Model file for the job. Use its own axes, mm. Face numbers are marked on the shaded views. A direction names the side the tool comes from. Round coordinates to 2 decimals unless told otherwise and drop trailing zeros. Loops run counter-clockwise (first coordinate to the right, second up) from the corner with the lowest first, then second, coordinate; pieces in that order, holes last. Notation, with made-up numbers: (44, 6) -> (70, 6) arc R14 cw to (70, 24) -> close; hole circle Ø7 at (58, 82). An arc over 180 degrees is marked (long way). Use a Markdown table: item, result.
from build123d import *

# Parameters (mm, degrees)
SKETCH_8_W      = 120
SKETCH_8_H      = 120
SKETCH_8_W_2    = 100
SKETCH_8_H_2    = 100
EXTRUDE_1_DEPTH = 225
SKETCH_9_W      = 160
SKETCH_9_H      = 160
SKETCH_9_R      = 25
EXTRUDE_2_DEPTH = 15
SKETCH_10_W     = 200
SKETCH_10_H     = 200
SKETCH_10_R     = 9
EXTRUDE_3_DEPTH = 20


with BuildPart() as part:
    # 草图8 → 凸台-拉伸1 (new, symmetric)
    with BuildSketch(Plane.XY):
        Rectangle(SKETCH_8_W, SKETCH_8_H)
        Rectangle(SKETCH_8_W_2, SKETCH_8_H_2, mode=Mode.SUBTRACT)
    extrude(amount=EXTRUDE_1_DEPTH, both=True)

    # 草图9 → 凸台-拉伸2 (add)
    with BuildSketch(Plane.XY.offset(225)):
        Rectangle(SKETCH_9_W, SKETCH_9_H)
        Circle(SKETCH_9_R, mode=Mode.SUBTRACT)
    extrude(amount=EXTRUDE_2_DEPTH)

    # 草图10 → 凸台-拉伸3 (add)
    with BuildSketch(Plane(origin=(0, 0, -225), x_dir=(-1, 0, 0), z_dir=(0, 0, -1))):
        Rectangle(SKETCH_10_W, SKETCH_10_H)
        with Locations((75, 75)):
            Circle(SKETCH_10_R, mode=Mode.SUBTRACT)
        with Locations((-75, 75)):
            Circle(SKETCH_10_R, mode=Mode.SUBTRACT)
        with Locations((75, -75)):
            Circle(SKETCH_10_R, mode=Mode.SUBTRACT)
        with Locations((-75, -75)):
            Circle(SKETCH_10_R, mode=Mode.SUBTRACT)
    extrude(amount=EXTRUDE_3_DEPTH)


solid = part.part
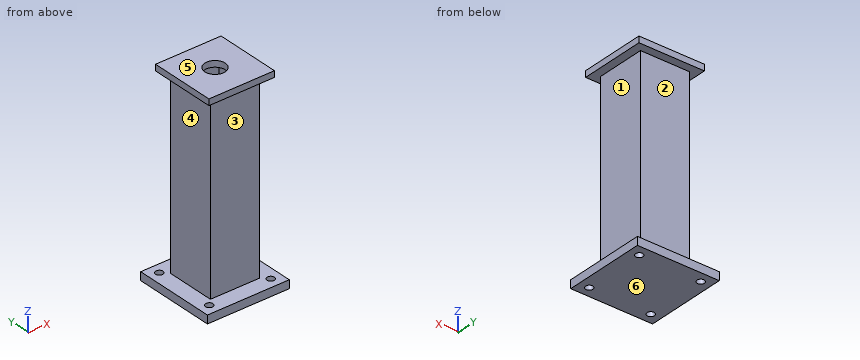
Q1. Band-saw the part on A-A, the plane z = 148. Give the cut face in (x, y).
Results list:
| item | result |
|---|---|
| outline | (-60, -60) -> (60, -60) -> (60, 60) -> (-60, 60) -> close; hole (-50, -50) -> (50, -50) -> (50, 50) -> (-50, 50) -> close |
Q2. Tool access for the marked faces 1, 2 and 3: list every direction of +Z, -Z, +X, -X, +Y, -Y with a clear straight run to the whole face (end or side of a thin tool).
Results list:
| item | result |
|---|---|
| face 1 | +X, +Y, -Y |
| face 2 | +X, -X, +Y |
| face 3 | +X, -X, -Y |
Q3. Band-saw the part on B-B, the plane x = -31.5. Give the cut face in (y, z).
Results list:
| item | result |
|---|---|
| outline | (-100, -245) -> (100, -245) -> (100, -225) -> (60, -225) -> (60, 225) -> (80, 225) -> (80, 240) -> (-80, 240) -> (-80, 225) -> (-60, 225) -> (-60, -225) -> (-100, -225) -> close; hole (-50, -225) -> (50, -225) -> (50, 225) -> (-50, 225) -> close |
Q4. Flat gauge pins, fed straight in: pin 1 (16.5 mm diameter, centred on x = -1.5, z = 230.5, fed in from +Y); pin 2 (11 mm diameter, centred on x = -75, y = 75, fed in from -Z); pin 3 (12 mm diameter, centred on x = -45, z = -89.5, fed in from +Y). Where does each tip first touch, or does it go through?
Results list:
| item | result |
|---|---|
| pin 1 | stops at y = 80 |
| pin 2 | stops at z = 225 |
| pin 3 | stops at y = 60 |
Q5. Pull direction Z, two halves, no side cores. Call the marked faces 4, 5 and 6: released by +Z, released by -Z, zero draft, split by the parting line, or undercut.
Results list:
| item | result |
|---|---|
| face 4 | undercut |
| face 5 | released by +Z |
| face 6 | released by -Z |
Q6. Band-saw the part on C-C, the plane y = 75. Give the cut face in (x, z).
Results list:
| item | result |
|---|---|
| outline | (-100, -245) -> (-84, -245) -> (-84, -225) -> (-100, -225) -> close; (-80, 225) -> (80, 225) -> (80, 240) -> (-80, 240) -> close; (-66, -245) -> (66, -245) -> (66, -225) -> (-66, -225) -> close; (84, -245) -> (100, -245) -> (100, -225) -> (84, -225) -> close |
Q7. Drill centre lines: L1, parallel to Y at x = 75, z = -235; L2, parallel to X at y = 22, z = -121. Where is each one in solid material? Low to high. Write a range as from..to.
Results list:
| item | result |
|---|---|
| L1 | y = -100..-84, -66..66, 84..100 |
| L2 | x = -60..-50, 50..60 |
